Part model, mm, in its own coordinate system. A direction names the side the tool comes from. Give positions to 0.01 mm unless a question says otherwise; leave off trailing zeros. Order: outer loops, then holes, each group sorted by start corner. A loop starts at its lowest first (then second) coordinate and runs counter-clockwise, first axis right, second up. Notation, with made-up numbers: (45, -26) - (82, -26) arc R19 ccw to (82, -8) - close; hole circle Ø6 at (46, -30.5). An arc over 180 degrees is marked (long way). One line per item, written item: value.
```python
from build123d import *

# Parameters (mm, degrees)
F1_DEPTH = 152.4
F2_DEPTH = 152.4
F4_DEPTH = 76.2


with BuildPart() as f1:
    # F0 (on Right) → F1 (new body)
    with BuildSketch(Plane.YZ):
        Polygon((-8.67072, 38.735581), (-34.07072, 38.735581), (-34.07072, -12.064419), (37.848741, -12.064419), (37.848741, 38.735581), (12.448741, 38.735581), (12.448741, 26.035581), (29.42928, 26.035581), (29.42928, 13.335581), (-21.37072, 13.335581), (-21.37072, 26.035581), (-8.67072, 26.035581), align=None)
    extrude(amount=-F1_DEPTH)

    # F0 (on Right) → F2 (join)
    with BuildSketch(Plane.YZ):
        Polygon((-8.67072, 38.735581), (-34.07072, 38.735581), (-34.07072, -12.064419), (37.848741, -12.064419), (37.848741, 38.735581), (12.448741, 38.735581), (12.448741, 26.035581), (29.42928, 26.035581), (29.42928, 13.335581), (-21.37072, 13.335581), (-21.37072, 26.035581), (-8.67072, 26.035581), align=None)
    extrude(amount=-F2_DEPTH)

    # F3 (on face) → F4 (cut)
    with BuildSketch(Plane.XZ.offset(34.07072)):
        Polygon((-125.592947, 0), (-113.217302, -12.064419), (-37.017302, -12.064419), (-23.992947, 0), align=None)
    extrude(amount=-F4_DEPTH, mode=Mode.SUBTRACT)


solid = f1.part
```
1) Mould opens along X. For faces 1 (the flat face through (-30.6, 1.39, -6.12)), 2 (the flat face through (-152.4, 1, 8)), 3 (the flat face through (0, 1, 8)), 4 (the flat face through (-75, 29.429, 20)) say: released by +X, released by -X, zero draft, split by the parting line, or undercut.
Outcome:
face 1: undercut
face 2: released by -X
face 3: released by +X
face 4: zero draft
2) Drill centre lines: line 1 along Z through (x, y) = (-118.5, 14.5); line 2 along Y through (x, z) = (-77, 17); line 3 along Z through (x, y) = (-83, -21). Where is each one in solid material? Low to high. Write a range as from..to.
Outcome:
line 1: z = -12.06..-6.91, 0..13.34, 26.04..38.74
line 2: y = -34.07..-21.37, 29.43..37.85
line 3: z = 0..13.34, 26.04..38.74
3) Cut at A-A, the plane z = 34. Give the cut face in (x, y), then the cut area to 3 significant figures.
Outcome:
outline: (-152.4, -34.07) - (0, -34.07) - (0, -8.67) - (-152.4, -8.67) - close; (-152.4, 12.45) - (0, 12.45) - (0, 37.85) - (-152.4, 37.85) - close
area: 7,740 mm^2
4) Cut at D-D, the plane y = -1.5. Give the cut face in (x, z), then the cut area to 3 significant figures.
Outcome:
outline: (-152.4, -12.06) - (-113.22, -12.06) - (-125.59, 0) - (-23.99, 0) - (-37.02, -12.06) - (0, -12.06) - (0, 13.34) - (-152.4, 13.34) - close
area: 2,800 mm^2
5) Cut at C-C, the plane x = -72. Give the cut face in (y, z).
Outcome:
outline: (-34.07, 0) - (37.85, 0) - (37.85, 38.74) - (12.45, 38.74) - (12.45, 26.04) - (29.43, 26.04) - (29.43, 13.34) - (-21.37, 13.34) - (-21.37, 26.04) - (-8.67, 26.04) - (-8.67, 38.74) - (-34.07, 38.74) - close
6) Pin check, flat tip, straight feed: pin 1 (4 mm diameter, centred on x = -43.5, y = -15.5, fed in from -Z). Stop position of the tip, or through.
Outcome:
pin 1: stops at z = 0
7) Cut at B-B, the plane y = 23. Give the cut face in (x, z).
Outcome:
outline: (-152.4, -12.06) - (-113.22, -12.06) - (-125.59, 0) - (-23.99, 0) - (-37.02, -12.06) - (0, -12.06) - (0, 13.34) - (-152.4, 13.34) - close; (-152.4, 26.04) - (0, 26.04) - (0, 38.74) - (-152.4, 38.74) - close
8) Which spindle directions (+Z, -Z, +X, -X, +Y, -Y) get a long thin tool onto all of the face, cutting with end or side? Do faces 5 (the flat face through (-75, -21.371, 20)), 6 (the flat face through (-74, 1, 0)), 7 (the flat face through (-75, 12.449, 32)). Say none if no direction does.
Outcome:
face 5: +X, -X
face 6: +Y, -Y
face 7: +Z, +X, -X
